Source: three-view drawing plus pictorial views. Frame: mm from the lowest corner of the part. A direction names the side the tool comes from. Coordinates: 2 decimals unless noted, no trailing zeros. Use CSV: the item, a comma, the result in double quotes. Start each with the question number.
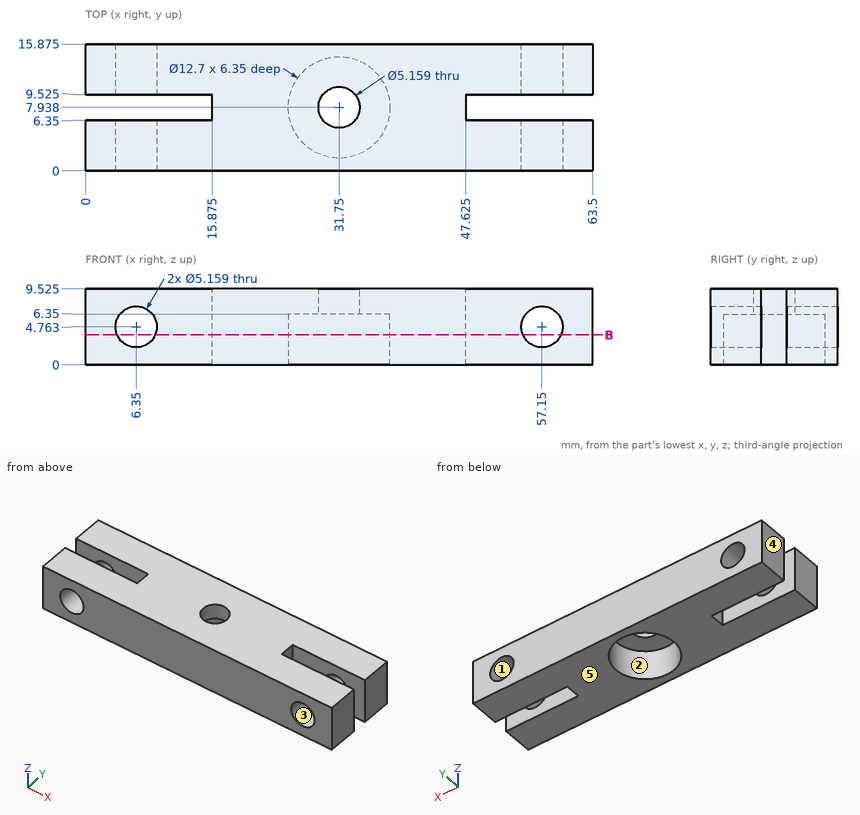
(1) Ray query, line 1 (X direction, y = 15.25, z = 4.5); line 2 (X direction, y = 13.5, z = 6.5) (1 decimal); line 3 (X direction, y = 5.25, z = 4) (1 decimal). Return the intervals inside material, ascending. Write a range as [from, to].
(2) Section B-B on z = 3.75. State how many separate pieces and enclosed holes the cut face has, plus the area to 3 significant figures.
(3) Pin query (flat end, axial travel): pin 1 Ø3 at (x, z) = (58, 6) entering from -Y; pin 2 Ø1 at (y, z) = (8, 5.5) entering from +X (1 decimal); pin 3 Ø4 at (x, y) = (29, 7) entering from -Z; pin 4 Ø1 at (y, z) = (8, 4) entering from -X (1 decimal). Return the tip coordinate at first contact, or that it passes through.
(4) Reachability of the marked faces 1 and 2 from +Z, -Z, +X, -X, +Y, -Y: full face, straight path, thin tool, end or side. Return the list, or none.
(5) Draft query along Z for the marked faces 3, 4 and 5. Return one class per face: released by +Z, released by -Z, zero draft, split by the parting line, or undercut.
Solution:
1,line 1,"x = [0, 3.78], [8.92, 54.58], [59.72, 63.5]"
1,line 2,"x = [0, 4.4], [8.3, 55.2], [59.1, 63.5]"
1,line 3,"x = [0, 3.9], [8.8, 26], [37.5, 54.7], [59.6, 63.5]"
2,separate pieces,"5"
2,enclosed holes,"1"
2,area,"660 mm²"
3,pin 1,"stops at y = 0"
3,pin 2,"stops at x = 47.6"
3,pin 3,"stops at z = 6.35"
3,pin 4,"stops at x = 15.9"
4,face 1,"+Y, -Y"
4,face 2,"-Z"
5,face 3,"undercut"
5,face 4,"zero draft"
5,face 5,"released by -Z"
